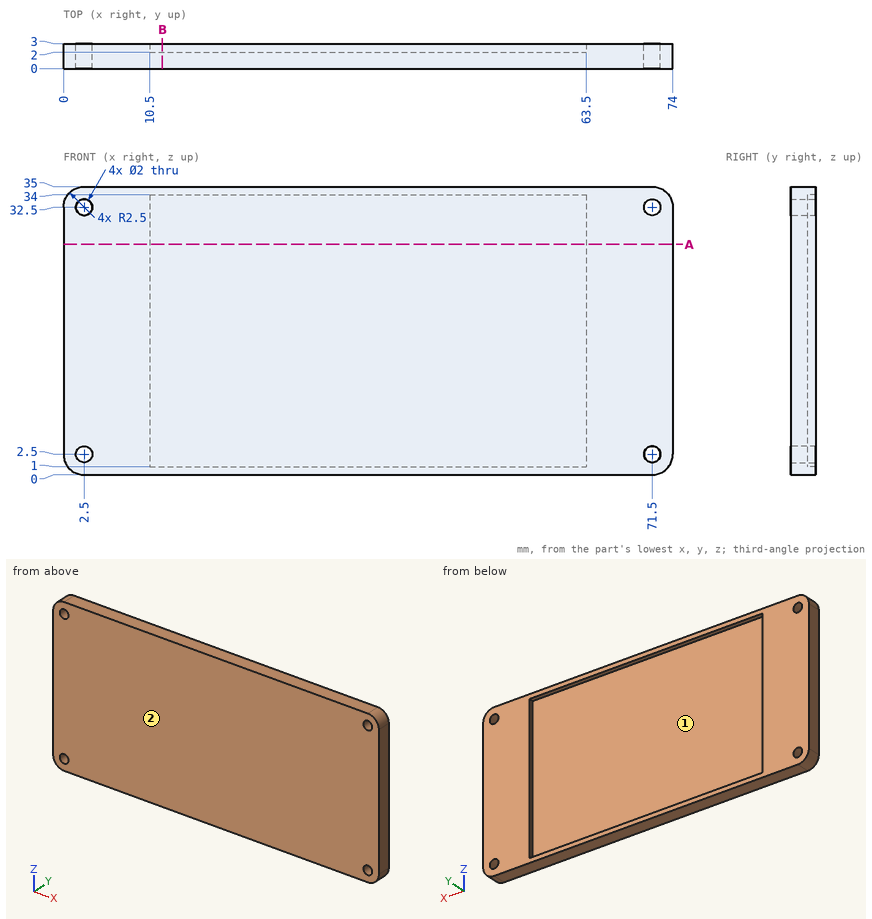
Could you check a few things on this drawing? It's one solid part, dimensions in mm from its lowest x, y, z. Give positions to 0.01 mm unless a question says otherwise; leave off trailing zeros. Order: outer loops, then holes, each group sorted by start corner. A loop starts at its lowest first (then second) coordinate and runs counter-clockwise, first axis right, second up. Notation, with made-up numbers: (12, 72.5) -> (49, 72.5) arc R22 ccw to (49, 90.5) -> close; hole circle Ø1 at (79.5, -17). An arc over 180 degrees is marked (long way). Use CSV: the item, a comma, the result in double quotes. Start each with the question number.
Item 1: Suppose I cut it at B-B (x = 12). List the corners of the cut face in (y, z) for me.
Item 2: Thinking about a two-plate mould opening in X: for the marked faces 1 and 2, which applies, pulls with the +X half, pulls with the -X half, needs draft (parallel to the pull), parting line crosses it, or undercut?
Item 3: Suppose I cut it at A-A (z = 28). List the corners of the cut face in (x, y) for me, and give its area (3 significant figures).
Item 4: I'm going to push a flat-ended pin straight in: P1, Ø16.5, axis at x = 49, z = 10.5, coming from the +Y side. Where does the tip first touch, or does it pass through?
Item 5: If I drill on probe 1 along Z at (x, y) = (2.5, 0.7); probe 2 along X at (y, z) = (1.8, 32.5); probe 3 along X at (y, z) = (2.3, 32.5), over which ranges is the centre line in solid material (lowest first)? Write a range as [from, to].
Answer block:
1,outline,"(0, 0) -> (3, 0) -> (3, 1) -> (2, 1) -> (2, 34) -> (3, 34) -> (3, 35) -> (0, 35) -> close"
2,face 1,"undercut"
2,face 2,"needs draft"
3,outline,"(0, 0) -> (74, 0) -> (74, 3) -> (63.5, 3) -> (63.5, 2) -> (10.5, 2) -> (10.5, 3) -> (0, 3) -> close"
3,area,"169 mm^2"
4,P1,"stops at y = 2"
5,probe 1,"z = [0, 1.5], [3.5, 31.5], [33.5, 35]"
5,probe 2,"x = [0, 1.5], [3.5, 70.5], [72.5, 74]"
5,probe 3,"x = [0, 1.5], [3.5, 10.5], [63.5, 70.5], [72.5, 74]"
